```python
from build123d import *

# Parameters (mm, degrees)
SKETCH1_W           = 25.4
SKETCH1_H           = 44.45
SKETCH1_R           = 9.525
BOSS_EXTRUDE1_DEPTH = 3.175
FILLET1_R           = 6.35


with BuildPart() as part:
    # Sketch1 → Boss-Extrude1 (new body)
    with BuildSketch(Plane.XY):
        with Locations((12.282474227, -21.155412371)):
            Rectangle(SKETCH1_W, SKETCH1_H)
        with Locations((12.035016268, -11.630412371)):
            Circle(SKETCH1_R, mode=Mode.SUBTRACT)
    extrude(amount=BOSS_EXTRUDE1_DEPTH)

    # Fillet1
    fillet1_edges = [part.edges().sort_by_distance(p)[0] for p in [
        (-0.417525773, 1.069587629, 1.5875),
        (24.982474227, 1.069587629, 1.5875),
    ]]
    fillet(fillet1_edges, radius=FILLET1_R)


solid = part.part
```
Could you check a few things on this model? Use its own coordinates, in mm. Give positions to 0.01 mm unless a question says otherwise; leave off trailing zeros. Write each loop counter-clockwise with the first axis right and the second up, starting at its lowest first coordinate (ties: lowest second). Pieces come first, ordered by that corner, then holes. Notation, with made-up numbers: (24, 26) - (33, 26) arc R32 ccw to (33, 58) - close; hole circle Ø3 at (-2.75, -39). An arc over 180 degrees is marked (long way). One line per item, written item: value. Start each with the question number.
Item 1: Imagine slicing it at D-D, the plane x = 23. List the corners of the cut face in (y, z) for me (3 decimals).
Item 2: Imagine slicing it at B-B, the plane y = -4.5. List the corners of the cut face in (x, z) for me (3 decimals).
Item 3: I'm going to push a flat-ended pin straight in: pin 1 (2 mm diameter, centred on x = 8.5, y = -19, fed in from +Z). Where does the tip first touch, or does it pass through?
Item 4: If we mould it in two halves opening along Y, with no side actions, what happens to faces 1 (the face through (12, -43.38, 2)), 2 (the face through (24.982, -25, 2)), 3 (the face through (21.12, -8.77, 1.57)), 4 (the face through (1.393, -0.84, 1.61))? For each: +Y half, -Y half, draft (parallel to the pull), parting line (faces both ways), or undercut.
Item 5: Please list where these lines run through material, in increasing order: line 1 (Y direction, x = 11.75, z = 0.25); line 2 (Y direction, x = 6, z = 2.75); line 3 (X direction, y = -18, z = 1.9). Write a range as from..to.
Item 6: Imagine slicing it at C-C, the plane z = 2.5. List the corners of the cut face in (x, y) for me (3 decimals), and give its area (3 significant figures).
Item 7: Imagine slicing it at A-A, the plane x = 15.25. List the corners of the cut face in (y, z) for me (3 decimals).
Geometry says:
1. outline: (-43.38, 0) - (-0.671, 0) - (-0.671, 3.175) - (-43.38, 3.175) - close
2. outline: (-0.369, 0) - (5.72, 0) - (5.72, 3.175) - (-0.369, 3.175) - close; (18.35, 0) - (24.934, 0) - (24.934, 3.175) - (18.35, 3.175) - close
3. pin 1: through
4. face 1: -Y half
4. face 2: draft
4. face 3: undercut
4. face 4: +Y half
5. line 1: -43.38..-21.15, -2.11..1.07
5. line 2: -43.38..-19, -4.26..1.07
5. line 3: -0.42..4.95, 19.12..24.98
6. outline: (-0.418, -43.38) - (24.982, -43.38) - (24.982, -5.28) arc R6.35 ccw to (18.632, 1.07) - (5.932, 1.07) arc R6.35 ccw to (-0.418, -5.28) - close; hole circle Ø19.05 at (12.035, -11.63)
6. area: 827 mm^2
7. outline: (-43.38, 0) - (-20.596, 0) - (-20.596, 3.175) - (-43.38, 3.175) - close; (-2.664, 0) - (1.07, 0) - (1.07, 3.175) - (-2.664, 3.175) - close
